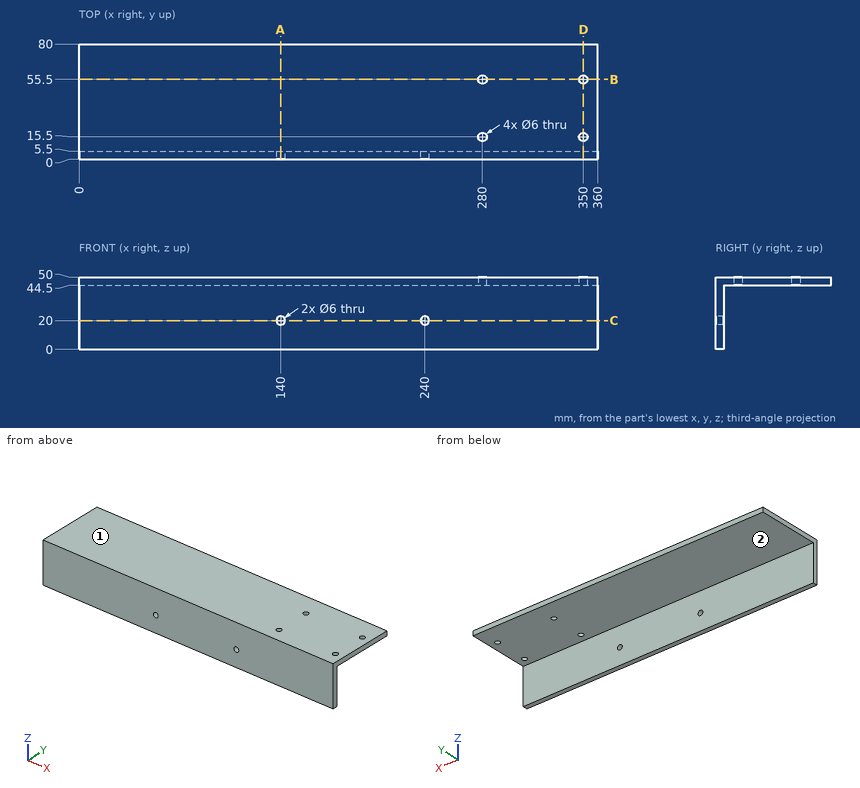
The figure shows three views and two pictorial views of one solid part (mm, origin at its lowest corner). Answer the questions. A direction names the side the tool comes from. Round coordinates to 2 decimals unless told otherwise and drop trailing zeros. Order: outer loops, then holes, each group sorted by start corner. A loop starts at its lowest first (then second) coordinate and runs counter-clockwise, first axis right, second up. Notation, with made-up numbers: M -14.5,75.5 L -0.5,75.5 A16 ccw -0.5,89.5 Z; hole C 77.25,36.5 d10. An arc over 180 degrees is marked long. Put each result on its own line as item: value. Start each with the question number.
Q1. Section D-D, the plane x = 350 is taken. Write down the section's boundary in (y, z).
Q2. Section B-B, the plane y = 55.5 is taken. Write down the section's boundary in (x, z).
Q3. A tool of negligible diameter and unlimited length cuts with its end or side. For the marked faces 1 and 2, from which of +Z, -Z, +X, -X, +Y, -Y can it reach the whole face along a straight path? Write none if from no direction.
Q4. Straight lines are drawn through the part: L1, parallel to Y at x = 350, z = 48; L2, parallel to X at y = 15.5, z = 48.05; L3, parallel to Z at x = 240, y = 3. For each, find the intervals that lie inside material, in ascending order. Write a range as [from, to].
Q5. Flat-ended cylindrical pins translate along their axes: pin 1 (1.5 mm diameter, centred on x = 84.5, y = 46.5, fed in from -Z); pin 2 (8 mm diameter, centred on x = 280, y = 15.5, fed in from +Z); pin 3 (22 mm diameter, centred on x = 161.5, z = 23, fed in from +Y). Find the tip coordinate at first contact, or state that the pin passes through.
Q6. Section C-C, the plane z = 20 is taken. Write down the section's boundary in (x, y).
Q7. Section A-A, the plane x = 140 is taken. Write down the section's boundary in (y, z), and give its area (3 significant figures).
Findings below:
1. outline: M 0,0 L 5.5,0 L 5.5,44.5 L 12.5,44.5 L 12.5,50 L 0,50 Z; M 18.5,44.5 L 52.5,44.5 L 52.5,50 L 18.5,50 Z; M 58.5,44.5 L 80,44.5 L 80,50 L 58.5,50 Z
2. outline: M 0,44.5 L 277,44.5 L 277,50 L 0,50 Z; M 283,44.5 L 347,44.5 L 347,50 L 283,50 Z; M 353,44.5 L 360,44.5 L 360,50 L 353,50 Z
3. face 1: +Z, +X, -X, +Y, -Y
3. face 2: -Z, +X, -X, +Y
4. L1: y = [0, 12.5], [18.5, 52.5], [58.5, 80]
4. L2: x = [0, 277], [283, 347], [353, 360]
4. L3: z = [0, 17], [23, 50]
5. pin 1: stops at z = 44.5
5. pin 2: stops at z = 50
5. pin 3: stops at y = 5.5
6. outline: M 0,0 L 137,0 L 137,5.5 L 0,5.5 Z; M 143,0 L 237,0 L 237,5.5 L 143,5.5 Z; M 243,0 L 360,0 L 360,5.5 L 243,5.5 Z
7. outline: M 0,0 L 5.5,0 L 5.5,17 L 0,17 Z; M 0,23 L 5.5,23 L 5.5,44.5 L 80,44.5 L 80,50 L 0,50 Z
7. area: 652 mm^2
